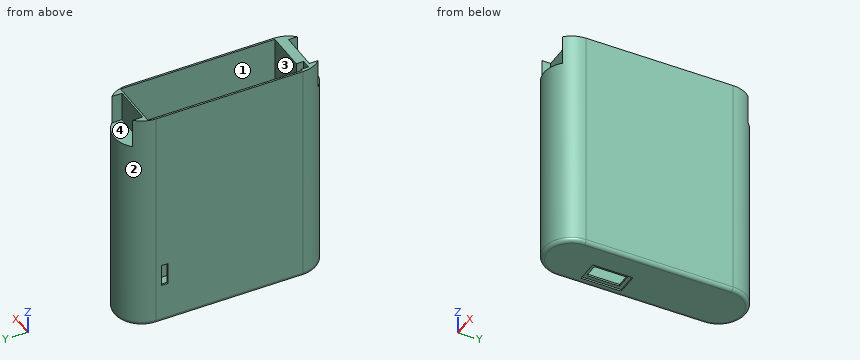
Autodesk Inventor part; units mm, degrees
ref_plane "YZ Plane" through (0, 0, 0) normal (1, 0, 0) x (0, 1, 0)
ref_plane "XZ Plane" through (0, 0, 0) normal (0, 1, 0) x (-1, 0, 0)
ref_plane "XY Plane" through (0, 0, 0) normal (0, 0, 1) x (1, 0, 0)
sketch "Boceto1" plane through (0, 0, 0) normal (0, 0, 1) x (1, 0, 0)
  line L0 (0, 0) -> (0, 40.1) construction
  line L1 (7.5, 0) -> (7.5, 40.1)
  line L2 (-7.5, 40.1) -> (-7.5, 0)
  arc A0 (-7.5, 0) -> (7.5, 0) centre (0, 0) ccw
  arc A1 (7.5, 40.1) -> (-7.5, 40.1) centre (0, 40.1) ccw
  point P0 (0, 20.05)
  dimension "d0" = 40.1
  dimension "d1" = 15
extrude "Extrusión1" add sketch "Boceto1" along normal blind 62
sketch "Boceto2" plane through (0, 0, 62) normal (0, 0, 1) x (1, 0, 0)
  line L0 (0, 0) -> (-7, 0)
  line L1 (-7, 0) -> (-7, 40.0875)
  line L2 (-7.5, 40.1) -> (-7.5, 0)
  line L3 (7, 0) -> (-7, 0)
  line L4 (-7, 40.0875) -> (-7, 42.1)
  arc A0 (7.5, 40.1) -> (-7.5, 40.1) centre (0, 40.1) ccw
  line L5 (-7, 42.1) -> (7, 42.1)
  line L6 (7, 42.1) -> (7, 0)
  dimension "d4" = 7
  dimension "d68" = 7
  dimension "d69" = 14
extrude "Extrusión2" cut sketch "Boceto2" against normal blind 61
sketch "Boceto3" plane through (0, 0, 62) normal (0, 0, 1) x (1, 0, 0)
  line L0 (-5.3571, -2.8499) -> (5.3571, -2.8499)
  line L1 (-6.5, 40.1) -> (6.5, 40.1)
  line L2 (-5, 42.6) -> (5, 42.6)
  line L3 (-5.3571, -2.8499) -> (-5.3571, -4.1499)
  line L4 (5.3571, -5.2489) -> (5.3571, -2.8499)
  arc A0 (7.5, 40.1) -> (-7.5, 40.1) centre (0, 40.1) ccw
  arc A1 (-5.3571, -5.2489) -> (5.3571, -5.2489) centre (0, 0) ccw
  line L5 (-5.3571, -4.1499) -> (-5.3571, -5.2489)
  arc A2 (-7.5, 0) -> (7.5, 0) centre (0, 0) ccw
  arc A3 (5.357, 45.3491) -> (-5.357, 45.3491) centre (0, 40.1) ccw
  line L6 (0, 42.6) -> (-5.357, 42.6)
  line L7 (-5.357, 42.6) -> (-5.357, 45.3491)
  line L8 (0, 42.6) -> (5.357, 42.6)
  line L9 (5.357, 42.6) -> (5.357, 45.3491)
  line L10 (0, -2.8499) -> (-5.357, -2.8499)
  point P0 (5.3571, -4.1499)
  point P1 (5, 43.9)
  dimension "d46" = 1.3
  dimension "d70" = 5.357
  dimension "d71" = 5.357
  dimension "d72" = 5.357
extrude "Extrusión3" cut sketch "Boceto3" against normal blind 8
fillet "Empalme1" radius 1 4 edges at (0, 47.6, 0) (-7.5, 20.05, 0) (0, -7.5, 0) (7.5, 20.05, 0)
sketch "Boceto5" plane through (0, 0, 62) normal (0, 0, 1) x (1, 0, 0)
  line L0 (7, 0) -> (-7, 0)
  line L1 (7, 0) -> (-3.5, 0)
  line L2 (5, -1) -> (-5, -1)
  line L3 (-3.5, -0.9) -> (-2, -0.9) construction
  arc A0 (-6.5, 0) -> (6.5, 0) centre (0, 0) ccw
  line L4 (-6.5, 0) -> (-3.5, 0)
  line L5 (-6.5, 0) -> (-6.5, -2)
  line L6 (-6.5, -2) -> (-5, -2)
  line L7 (-5, -2) -> (-4, -2)
  line L8 (-4, -2) -> (-4, 0)
  line L9 (7, 0) -> (-7, 0)
  dimension "d49" = 2
  dimension "d51" = 1
extrude "Extrusión5" cut sketch "Boceto5" against normal blind 60 contours L6 L5 A0 | A0 L0 L8 L7 L6 picked at (-5.1549, -1.2255)
sketch "Boceto6" plane through (0, 0, 0) normal (0, 0, -1) x (-1, 0, 0)
  line L0 (-7, 0) -> (7, 0)
  line L1 (3.5, 0) -> (3.5, 6.5)
  line L2 (6.5, 40.1) -> (-6.5, 40.1)
  line L3 (-0.5, 0) -> (3.5, 0)
  line L4 (7, 0) -> (7, 42.1)
  line L5 (6.5, 40.1) -> (6.5, 0)
  line L6 (4.5, 6.5) -> (4.5, 15.5)
  line L7 (4.5, 15.5) -> (0.5, 15.5)
  line L8 (0.5, 15.5) -> (0.5, 6.5)
  line L9 (-0.5, 0) -> (0.5, 0)
  line L10 (-7, 0) -> (7, 0)
  line L11 (0.5, 0) -> (0.5, 6.5)
  line L12 (4.5, 6.5) -> (0.5, 6.5)
  point P0 (0, 0)
  point P1 (7, 42.1)
  dimension "d44" = 9
  dimension "d60" = 1
extrude "Extrusión6" cut sketch "Boceto6" against normal through all contours L8 L7 L6 L12
sketch "Boceto7" plane through (-7.5, 0, 62) normal (-1, 0, 0) x (0, 0, 1)
  line L0 (-45, 36.8) -> (-45, 38.6)
  line L1 (-45, 38.6) -> (-51, 38.6)
  line L2 (-51, 38.6) -> (-51, 36.8)
  line L3 (-51, 36.8) -> (-45, 36.8)
  point P0 (-62, 0)
  dimension "d74" = 6
extrude "Extrusión7" cut sketch "Boceto7" against normal blind 3
sketch "Boceto8" plane through (0, 0, 0) normal (0, 0, -1) x (-1, 0, 0)
  line L0 (0.5, 6.5) -> (0.5, 15.5)
  line L1 (4.5, 15.5) -> (4.5, 6.5)
  line L2 (0.5, 15.5) -> (4.5, 15.5)
  line L3 (4.5, 15.5) -> (4.5, 6.5)
  line L4 (4.5, 6.5) -> (0.5, 6.5)
  line L5 (0.5, 6.5) -> (0.5, 15.5)
  line L6 (5.5, 16.5) -> (-0.5, 16.5)
  line L7 (-0.5, 16.5) -> (-0.5, 5.5)
  line L8 (-0.5, 5.5) -> (5.5, 5.5)
  line L9 (5.5, 5.5) -> (5.5, 16.5)
  point P0 (0, 0)
  dimension "d61" = 1
extrude "Extrusión8" cut sketch "Boceto8" against normal blind 0.5 contours L0 L2 L1 L4 | L9 L8 L7 L6
sketch "Boceto9" plane through (-7.5, 0, 62) normal (-1, 0, 0) x (0, 0, 1)
  point P0 (-62, 0)
properties part number "Carcasa Luis"
Could you check a few things on this model? Use its own coordinates, in mm. Face numbers are marked on the shaded views. Round coordinates to 2 decimals unless told otherwise and drop trailing zeros. Loops run counter-clockwise (first coordinate to the right, second up) from the corner with the lowest first, then second, coordinate; pieces in that order, holes last. Notation, with made-up numbers: M 50,-8.75 L 76,-8.75 A19 ccw 76,9.25 Z; hole C 23,-20 d10. An arc over 180 degrees is marked long. Put each result on its own line as item: value.
Q1. Thinking about a two-plate mould opening in Y: for the marked faces 1, 2, 3 and 4, which applies, released by +Y, released by -Y, zero draft, split by the parting line, or undercut?
Check result:
face 1: undercut
face 2: released by +Y
face 3: undercut
face 4: zero draft
Q2. I need wall thicknesses on probe 1 along X at (y, z) = (9.5, 25.5); probe 2 along Y at (x, z) = (-3.25, 59); probe 3 along Y at (x, z) = (-3.75, 46). Which ranges of each line are inside material? Lowest first, please.
Check result:
probe 1: -7.5 to -7, 7 to 7.5
probe 2: -2.85 to 0, 42.1 to 42.6
probe 3: -6.5 to 0, 42.1 to 46.6
Q3. Imagine slicing it at B-B (z = 30). Write out the boundary of the cut face in (x, y), then the cut area to 3 significant figures.
Check result:
outline: M -7.5,0 A7.5 ccw 7.5,0 L 7.5,40.1 A7.5 ccw -7.5,40.1 Z; hole M -7,0 L -6.5,0 L -6.5,-2 L -4,-2 L -4,0 L 7,0 L 7,42.1 L -7,42.1 Z
area: 184 mm2
Q4. For pin 1 (1 mm diameter, centred on y = -1.5, z = 42.5, fed in from -X); pin 2 (1.4 mm diameter, centred on y = 44, z = 59, fed in from -X); pin 3 (1.9 mm diameter, centred on y = -4.5, z = 60, fed in from +X), each with a flat end and sliding along its axis, tell me the tip position at first contact or that it passes through.
Check result:
pin 1: x = -7.43
pin 2: x = -6.78
pin 3: x = 6.61
Q5. Imagine slicing it at A-A (y = 13). Write out the boundary of the cut face in (x, z).
Check result:
outline: M -7.5,1 A1 ccw -6.5,0 L -5.5,0 L -5.5,0.5 L -4.5,0.5 L -4.5,1 L -7,1 L -7,62 L -7.5,62 Z; M -0.5,0.5 L 0.5,0.5 L 0.5,0 L 6.5,0 A1 ccw 7.5,1 L 7.5,62 L 7,62 L 7,1 L -0.5,1 Z
Q6. Imagine slicing it at C-C (y = 35.5). Write out the boundary of the cut face in (x, z).
Check result:
outline: M -7.5,1 A1 ccw -6.5,0 L 6.5,0 A1 ccw 7.5,1 L 7.5,62 L 7,62 L 7,1 L -7,1 L -7,62 L -7.5,62 Z
